Input: part model. Units: mm. Frame: model coordinates. A direction names the side the tool comes from. Round coordinates to 2 decimals unless told otherwise and drop trailing zeros. Loops run counter-clockwise (first coordinate to the right, second up) from the corner with the lowest first, then second, coordinate; pieces in that order, holes last. Notation, with made-up numbers: M 81.25,35.25 L 88.25,35.25 A27 cw 88.25,70.25 Z; hole C 73,83.25 d11. An arc over 180 degrees is marked long. Return JSON: item names as keys, results as strings. Group by question number.
1) Material intervals for line 1 (X direction, y = -14.5, z = 61.05); line 2 (X direction, y = -1, z = -22); line 3 (Y direction, x = 72.5, z = 60.75), sorted ascending. Write a range as from..to.
2) Section C-C (z = -65). Output: boundary loops of the cut face in (x, y).
3) Mould query, pull axis X, two halves, no side actions, for faces 1 (the face through (-115, -1, 5)), 2 (the face through (-80, -30, 62)), 3 (the face through (45, -1, -33)). Classes: +X half, -X half, draft (parallel to the pull), parting line (faces both ways), or undercut.
4) Section A-A (x = 80). Output: boundary loops of the cut face in (y, z), plus the area to 3 significant figures.
5) Section B-B (y = -51). Output: boundary loops of the cut face in (x, z), plus the area to 3 significant figures.
6) Section D-D (z = 22.5). Output: boundary loops of the cut face in (x, y), plus the area to 3 significant figures.
7) Contact query for flat-ended pins moving along their axis: P1, Ø1.6, axis at x = -168, y = -1, coming from the +Z side; P2, Ø9.5, axis at x = 80, z = -79, coming from the -Y side; P3, Ø0.6, axis at y = -0.5, z = -82.5, coming from the -X side; P4, Ø12, axis at x = 1, y = -9.5, coming from the +Z side. Output: stop coordinate, or through.
8) Access query for faces 4 (the face through (-50, -24, 61)), 5 (the face through (-81.8, -1, -81.4)), 6 (the face through (-55, -1, -94)), 7 (the face through (80, -30, 60)). Directions: +Z, -Z, +X, -X, +Y, -Y. A direction counts if a zero-diameter tool reaches every point of the face in a straight line with its end or side. Return the directions, or none.
from build123d import *

# Parameters (mm, degrees)
SM_BASE_FLANGE_1_DEPTH            = 2
SM_EDGE_FLANGE_2_STRIP_W          = 10
SM_EDGE_FLANGE_2_STRIP_H          = 2
SM_EDGE_FLANGE_2_STRIP_CUT_DEPTH  = 220
SM_EDGE_FLANGE_2_RELIEF_W         = 11
SM_EDGE_FLANGE_2_RELIEF_H         = 1
SM_EDGE_FLANGE_2_RELIEF_CUT_DEPTH = 2
SM_EDGE_FLANGE_2_DEPTH            = 220
CUT_EXTRUDE_START                 = 62
SKETCH_12_R                       = 2
CUT_EXTRUDE_4_DEPTH               = 2
SKETCH_14_R                       = 2
CUT_EXTRUDE_2_DEPTH               = 2
SKETCH_15_W                       = 100
SKETCH_15_H                       = 25
CUT_EXTRUDE_3_DEPTH               = 57
SKETCH_16_W                       = 100
SKETCH_16_H                       = 60
CUT_EXTRUDE_6_DEPTH               = 2
CUT_EXTRUDE_START_2               = -2
SKETCH_18_R                       = 3
CUT_EXTRUDE_7_DEPTH               = 2
OTHER_START                       = -2
OTHER_2_DEPTH                     = 2
SKETCH_20_W                       = 60
SKETCH_20_H                       = 61
CUT_EXTRUDE_8_DEPTH               = 2
SKETCH_21_R                       = 3
CUT_EXTRUDE_9_DEPTH               = 2
OTHER_4_DEPTH                     = 2
OTHER_4_2_DEPTH                   = 2


# Read off the part's stored shape, not the designer's step: 断开-边角2, 断开-边角4
# Sheet-metal steps are written as plain solids
with BuildPart() as part:
    # Sketch 1 → 基体-法兰1 (new body)
    with BuildSketch(Plane(origin=(0, 0, 0), x_dir=(1, 0, 0), z_dir=(0, 1, 0))):
        Polygon((-110, -60), (110, -60), (110, 60), (110, 160), (-110, 160), (-110, 60), (-210, 60), (-210, -60), align=None)
    extrude(amount=-SM_BASE_FLANGE_1_DEPTH)

    # 边线-法兰2 strip (across the edge) → 边线-法兰2 strip cut (cut)
    with BuildSketch(Plane(origin=(110, -2, 60), x_dir=(0, 0, -1), z_dir=(-1, 0, 0))):
        with Locations((-4, -1)):
            Rectangle(SM_EDGE_FLANGE_2_STRIP_W, SM_EDGE_FLANGE_2_STRIP_H)
    extrude(amount=SM_EDGE_FLANGE_2_STRIP_CUT_DEPTH, mode=Mode.SUBTRACT)

    # 边线-法兰2 relief (on the sheet) → 边线-法兰2 relief cut (cut)
    with BuildSketch(Plane(origin=(110, -2, 59), x_dir=(0, 0, -1), z_dir=(0, -1, 0))):
        with Locations((-4.5, -220.5)):
            Rectangle(SM_EDGE_FLANGE_2_RELIEF_W, SM_EDGE_FLANGE_2_RELIEF_H)
    extrude(amount=-SM_EDGE_FLANGE_2_RELIEF_CUT_DEPTH, mode=Mode.SUBTRACT)

    # 边线-法兰2 section (across the edge) → 边线-法兰2 (add)
    with BuildSketch(Plane(origin=(110, -2, 60), x_dir=(0, 0, -1), z_dir=(-1, 0, 0))):
        with BuildLine():
            Line((-2, 1), (-2, 55))
            Line((-2, 55), (0, 55))
            Line((0, 55), (0, 1))
            ThreePointArc((0, 1), (0.292893219, 0.292893219), (1, 0))
            Line((1, 0), (1, -2))
            ThreePointArc((1, -2), (-1.121320344, -1.121320344), (-2, 1))
        make_face()
    extrude(amount=SM_EDGE_FLANGE_2_DEPTH)

    # 草图12 → 切除-拉伸4 (cut)
    with BuildSketch(Plane.XY.offset(CUT_EXTRUDE_START)):
        with Locations(Location((72.5, -14.5, 0), (0, 0, 90))):
            Circle(SKETCH_12_R)
        with Locations(Location((-77.5, -14.5, 0), (0, 0, 90))):
            Circle(SKETCH_12_R)
        with Locations(Location((-77.5, -39.5, 0), (0, 0, 90))):
            Circle(SKETCH_12_R)
        with Locations(Location((72.5, -39.5, 0), (0, 0, 90))):
            Circle(SKETCH_12_R)
    extrude(amount=-CUT_EXTRUDE_4_DEPTH, mode=Mode.SUBTRACT)

    # 草图14 → 切除-拉伸2 (cut)
    with BuildSketch(Plane(origin=(0, 0, 0), x_dir=(1, 0, 0), z_dir=(0, 1, 0))):
        with Locations(Location((-77.5, 22.5, 0), (0, 0, 270))):
            Circle(SKETCH_14_R)
        with Locations(Location((-77.5, -27.5, 0), (0, 0, 270))):
            Circle(SKETCH_14_R)
        with Locations(Location((72.5, 22.5, 0), (0, 0, 270))):
            Circle(SKETCH_14_R)
        with Locations(Location((72.5, -27.5, 0), (0, 0, 270))):
            Circle(SKETCH_14_R)
    extrude(amount=-CUT_EXTRUDE_2_DEPTH, mode=Mode.SUBTRACT)

    # 草图15 → 切除-拉伸3 (cut)
    with BuildSketch(Plane(origin=(0, 0, 0), x_dir=(1, 0, 0), z_dir=(0, 1, 0))):
        with Locations((0, -49.5)):
            Rectangle(SKETCH_15_W, SKETCH_15_H)
        Polygon((-50, 53), (-50, 28), (50, 28), (50, 53), (50, 160), (-50, 160), align=None)
    extrude(amount=-CUT_EXTRUDE_3_DEPTH, mode=Mode.SUBTRACT)

    # 草图16 → 切除-拉伸6 (cut)
    with BuildSketch(Plane(origin=(0, 0, 0), x_dir=(1, 0, 0), z_dir=(0, 1, 0))):
        with Locations((-160, -30)):
            Rectangle(SKETCH_16_W, SKETCH_16_H)
    extrude(amount=-CUT_EXTRUDE_6_DEPTH, mode=Mode.SUBTRACT)

    # 草图18 → 切除-拉伸7 (cut)
    with BuildSketch(Plane(origin=(0, 0, 0), x_dir=(1, 0, 0), z_dir=(0, 1, 0)).offset(CUT_EXTRUDE_START_2)):
        with Locations(Location((-80, 140, 0), (0, 0, 270))):
            Circle(SKETCH_18_R)
        with Locations(Location((80, 140, 0), (0, 0, 270))):
            Circle(SKETCH_18_R)
        with Locations(Location((-190, 30, 0), (0, 0, 270))):
            Circle(SKETCH_18_R)
    extrude(amount=CUT_EXTRUDE_7_DEPTH, mode=Mode.SUBTRACT)

    # Other 2 outline → Other 2 (add)
    with BuildSketch(Plane(origin=(0, 0, 0), x_dir=(1, 0, 0), z_dir=(0, 1, 0)).offset(OTHER_START)):
        Polygon((-50, -37), (-50, -47), (-40, -37), align=None)
        Polygon((50, -37), (40, -37), (50, -47), align=None)
        Polygon((50, 28), (50, 38), (40, 28), align=None)
        Polygon((-50, 28), (-40, 28), (-50, 38), align=None)
    extrude(amount=OTHER_2_DEPTH)

    # 草图20 → 切除-拉伸8 (cut)
    with BuildSketch(Plane(origin=(0, 0, 0), x_dir=(1, 0, 0), z_dir=(0, 1, 0))):
        with Locations((-80, 129.5)):
            Rectangle(SKETCH_20_W, SKETCH_20_H)
        with Locations((80, 129.5)):
            Rectangle(SKETCH_20_W, SKETCH_20_H)
    extrude(amount=-CUT_EXTRUDE_8_DEPTH, mode=Mode.SUBTRACT)

    # 草图21 → 切除-拉伸9 (cut)
    with BuildSketch(Plane(origin=(0, 0, 0), x_dir=(1, 0, 0), z_dir=(0, 1, 0))):
        with Locations(Location((-80, 79, 0), (0, 0, 270))):
            Circle(SKETCH_21_R)
        with Locations(Location((80, 79, 0), (0, 0, 270))):
            Circle(SKETCH_21_R)
    extrude(amount=-CUT_EXTRUDE_9_DEPTH, mode=Mode.SUBTRACT)

    # Other 4 outline → Other 4 (cut)
    with BuildSketch(Plane(origin=(0, 0, 0), x_dir=(1, 0, 0), z_dir=(0, 1, 0)).offset(OTHER_START)):
        Polygon((-50, 99), (-60, 99), (-50, 89), align=None)
        Polygon((-200, 0), (-210, 10), (-210, 0), align=None)
        Polygon((-210, 50), (-200, 60), (-210, 60), align=None)
        Polygon((-110, 89), (-100, 99), (-110, 99), align=None)
        Polygon((50, 99), (50, 89), (60, 99), align=None)
        Polygon((110, 99), (100, 99), (110, 89), align=None)
    extrude(amount=OTHER_4_DEPTH, mode=Mode.SUBTRACT)

    # Other 4 2 outline → Other 4 2 (add)
    with BuildSketch(Plane(origin=(0, 0, 0), x_dir=(1, 0, 0), z_dir=(0, 1, 0)).offset(OTHER_START)):
        Polygon((-110, 0), (-120, 0), (-110, -10), align=None)
        Polygon((-110, 60), (-110, 70), (-120, 60), align=None)
    extrude(amount=OTHER_4_2_DEPTH)


solid = part.part
Returned:
{
 "1": {"line 1": "x = -110..-79.5, -75.5..-50, 50..70.5, 74.5..110", "line 2": "x = -210..-79.44, -75.56..70.56, 74.44..110", "line 3": "y = -57..-41.5, -37.5..-16.5, -12.5..-0.56"},
 "2": {"outline": "M -115,-2 L -50,-2 L -50,0 L -115,0 Z; M 50,-2 L 110,-2 L 110,0 L 50,0 Z"},
 "3": {"face 1": "-X half", "face 2": "draft", "face 3": "undercut"},
 "4": {"outline": "M -57,60 L -3,60 A1 cw -2,59 L -2,-76 L 0,-76 L 0,59 A3 ccw -3,62 L -57,62 Z; M -2,-99 L 0,-99 L 0,-82 L -2,-82 Z", "area": "418 mm^2"},
 "5": {"outline": "M -110,60 L -50,60 L -50,62 L -110,62 Z; M 50,60 L 110,60 L 110,62 L 50,62 Z", "area": "240 mm^2"},
 "6": {"outline": "M -110,-2 L 110,-2 L 110,0 L -110,0 Z", "area": "440 mm^2"},
 "7": {"P1": "stops at z = 0", "P2": "stops at y = -2", "P3": "stops at x = -110", "P4": "passes through"},
 "8": {"face 4": "+Z, +Y, -Y", "face 5": "+Y, -Y", "face 6": "-Z, +Y, -Y", "face 7": "-Z, +X, -X, -Y"}
}
